Input: part model. Units: mm. Frame: model coordinates. A direction names the side the tool comes from. Coordinates: 2 decimals unless noted, no trailing zeros. Order: outer loops, then holes, each group sorted by start corner. A loop starts at its lowest first (then second) coordinate and runs counter-clockwise, first axis right, second up. Notation, with made-up numbers: (-3.5, -30.75) - (18.5, -30.75) arc R21 cw to (18.5, -8.75) - close; hole circle Ø10 at (-2.5, -15). An arc over 180 degrees is marked (long way). Answer as CSV lines item,"result". Start each with the question number.
Item 1: First-contact query: pin 1 (19.5 mm diameter, centred on x = 8.5, y = 0.5, fed in from +Z); pin 2 (6 mm diameter, centred on x = -6, z = -6.5, fed in from +Y); pin 3 (5 mm diameter, centred on x = -67, y = 35, fed in from +Z). Flat tips, straight axial feed; report the tip coordinate or a pass-through.
Item 2: Draft query along Y for faces 4 (the flat face through (0, 0, -40)), 5 (the flat face through (-1, -100, 20)), 6 (the flat face through (-1, 97, 21)). Return one class per face: +Y half, -Y half, draft (parallel to the pull), parting line (faces both ways), or undercut.
Item 3: Access query for faces 1 (the flat face through (-100, -1, 20)), 2 (the flat face through (0, 0, -37)), 3 (the cylindrical face through (10.382, -19.961, -19.72)). Directions: +Z, -Z, +X, -X, +Y, -Y. A direction counts if a zero-diameter tool reaches every point of the face in a straight line with its end or side. Return the directions, or none.
Item 4: Section B-B (x = 62.5). Output: boundary loops of the cut face in (y, z).
Item 5: Section D-D (x = 0). Output: boundary loops of the cut face in (y, z), and give its area (3 significant figures).
Item 6: Section A-A (z = 15). Output: boundary loops of the cut face in (x, y).
Item 7: Material intervals for line 1 along Y through (x, z) = (35.5, 36.5); line 2 along Y through (x, z) = (0, -18); line 3 along Z through (x, y) = (88, -49.5), sorted ascending.
from build123d import *

# Parameters (mm, degrees)
SKETCH_1_W      = 200
SKETCH_1_H      = 200
EXTRUDE_1_DEPTH = 40
SKETCH_2_R      = 22.5
EXTRUDE_2_DEPTH = 40
SHELL_1_T       = -3


with BuildPart() as part:
    # ｽｹｯﾁ1 → ﾎﾞｽ - 押し出し1 (new body)
    with BuildSketch(Plane.XY):
        Rectangle(SKETCH_1_W, SKETCH_1_H)
    extrude(amount=EXTRUDE_1_DEPTH)

    # ｽｹｯﾁ2 → ﾎﾞｽ - 押し出し2 (add)
    with BuildSketch(Plane.XY):
        Circle(SKETCH_2_R)
    extrude(amount=-EXTRUDE_2_DEPTH)

    # ｼｪﾙ1
    shell_1_openings = [part.faces().sort_by_distance(p)[0] for p in [
        (0, 0, 40),
    ]]
    offset(amount=SHELL_1_T, openings=shell_1_openings, kind=Kind.INTERSECTION)


solid = part.part
Determined:
1,pin 1,"stops at z = -37"
1,pin 2,"stops at y = 22.3"
1,pin 3,"stops at z = 3"
2,face 4,"draft"
2,face 5,"-Y half"
2,face 6,"undercut"
3,face 1,"+Z, -Z, -X, +Y, -Y"
3,face 2,"+Z"
3,face 3,"-Z"
4,outline,"(-100, 0) - (100, 0) - (100, 40) - (97, 40) - (97, 3) - (-97, 3) - (-97, 40) - (-100, 40) - close"
5,outline,"(-100, 0) - (-22.5, 0) - (-22.5, -40) - (22.5, -40) - (22.5, 0) - (100, 0) - (100, 40) - (97, 40) - (97, 3) - (19.5, 3) - (19.5, -37) - (-19.5, -37) - (-19.5, 3) - (-97, 3) - (-97, 40) - (-100, 40) - close"
5,area,"1,060 mm^2"
6,outline,"(-100, -100) - (100, -100) - (100, 100) - (-100, 100) - close; hole (-97, -97) - (97, -97) - (97, 97) - (-97, 97) - close"
7,line 1,"y = -100 to -97, 97 to 100"
7,line 2,"y = -22.5 to -19.5, 19.5 to 22.5"
7,line 3,"z = 0 to 3"
